Verification items for the finished model (mm, model axes). Give positions to 0.01 mm unless a question says otherwise; leave off trailing zeros. Order: outer loops, then holes, each group sorted by start corner. A loop starts at its lowest first (then second) coordinate and runs counter-clockwise, first axis right, second up. Notation, with made-up numbers: (8, -34) -> (66, -34) arc R18 ccw to (66, -16) -> close; hole circle Ø4 at (-24.75, 62). An arc over 180 degrees is marked (long way). Return JSON: item names as keys, results as strings. Group by question number.
(1) Depth check by flat-ended pin: pin 1 Ø2.5 at (x, y) = (-42.57, 10.96) entering from +Z. Enter the tip coordinate at first touch or a pass-through.
(2) Release check for a two-part mould opening along Y. For faces 1 (the face through (-52.416, -40.555, 1.479)), 2 (the face through (20.33, 73.54, 1.48)), 3 (the face through (20.24, -42.79, 1.48)) record: pulls with the +Y half, pulls with the -Y half, needs draft (parallel to the pull), parting line crosses it, or undercut.
(3) Thickness scan on line 1 along Y through (x, z) = (14.5, 2.65); line 2 along X through (y, z) = (54.5, 0.3); line 3 along Y through (x, z) = (-53.5, 1.9). Record the ranges inside material, lowest first.
(4) Cross-section at A-A on x = 7.5. Enter the section's corners in (y, z).
from build123d import *

# Parameters (mm, degrees)
IZIM1_R                     = 2.1
Y_KSEKLIK_EKSTR_ZYON1_DEPTH = 3
IZIM2_R                     = 2.1
KES_EKSTR_ZYON1_DEPTH       = 10


with BuildPart() as part:
    # Çizim1 → Yükseklik-Ekstrüzyon1 (new body)
    with BuildSketch(Plane.XY):
        with BuildLine():
            Line((22.039642989, -38.504590939), (22.039642989, 69.347448082))
            ThreePointArc((22.039642989, 69.347448082), (20.282283676, 73.590088769), (16.039642989, 75.347448082))
            Line((16.039642989, 75.347448082), (-51.960357011, 75.347448082))
            ThreePointArc((-51.960357011, 75.347448082), (-56.202997698, 73.590088769), (-57.960357011, 69.347448082))
            Line((-57.960357011, 69.347448082), (-57.960357011, -38.504590939))
            ThreePointArc((-57.960357011, -38.504590939), (-56.202997698, -42.747231626), (-51.960357011, -44.504590939))
            Line((-51.960357011, -44.504590939), (16.039642989, -44.504590939))
            ThreePointArc((16.039642989, -44.504590939), (20.282283676, -42.747231626), (22.039642989, -38.504590939))
        make_face()
        with Locations((-51.960357011, -38.504590939)):
            Circle(IZIM1_R, mode=Mode.SUBTRACT)
        with Locations((16.039642989, -38.504590939)):
            Circle(IZIM1_R, mode=Mode.SUBTRACT)
        with Locations((16.039642989, 69.347448082)):
            Circle(IZIM1_R, mode=Mode.SUBTRACT)
        with Locations((-51.960357011, 69.347448082)):
            Circle(IZIM1_R, mode=Mode.SUBTRACT)
    extrude(amount=Y_KSEKLIK_EKSTR_ZYON1_DEPTH)

    # Çizim2 → Kes-Ekstrüzyon1 (cut)
    with BuildSketch(Plane(origin=(0, 0, 0), x_dir=(-1, 0, 0), z_dir=(0, 0, -1))):
        with Locations((17.960357011, 53.578572425)):
            Circle(IZIM2_R)
        with Locations((42.568052166, 10.95679416)):
            Circle(IZIM2_R)
        with Locations((-6.647338144, 10.95679416)):
            Circle(IZIM2_R)
    extrude(amount=-KES_EKSTR_ZYON1_DEPTH, mode=Mode.SUBTRACT)


solid = part.part
Verdict:
{
 "1": {"pin 1": "through"},
 "2": {"face 1": "undercut", "face 2": "pulls with the +Y half", "face 3": "pulls with the -Y half"},
 "3": {"line 1": "-44.5 to -39.93, -37.08 to 67.92, 70.78 to 75.35", "line 2": "-57.96 to -19.85, -16.07 to 22.04", "line 3": "-44.3 to -39.93, -37.08 to 67.92, 70.78 to 75.15"},
 "4": {"outline": "(-44.5, 0) -> (9.04, 0) -> (9.04, 3) -> (-44.5, 3) -> close; (12.88, 0) -> (75.35, 0) -> (75.35, 3) -> (12.88, 3) -> close"}
}
